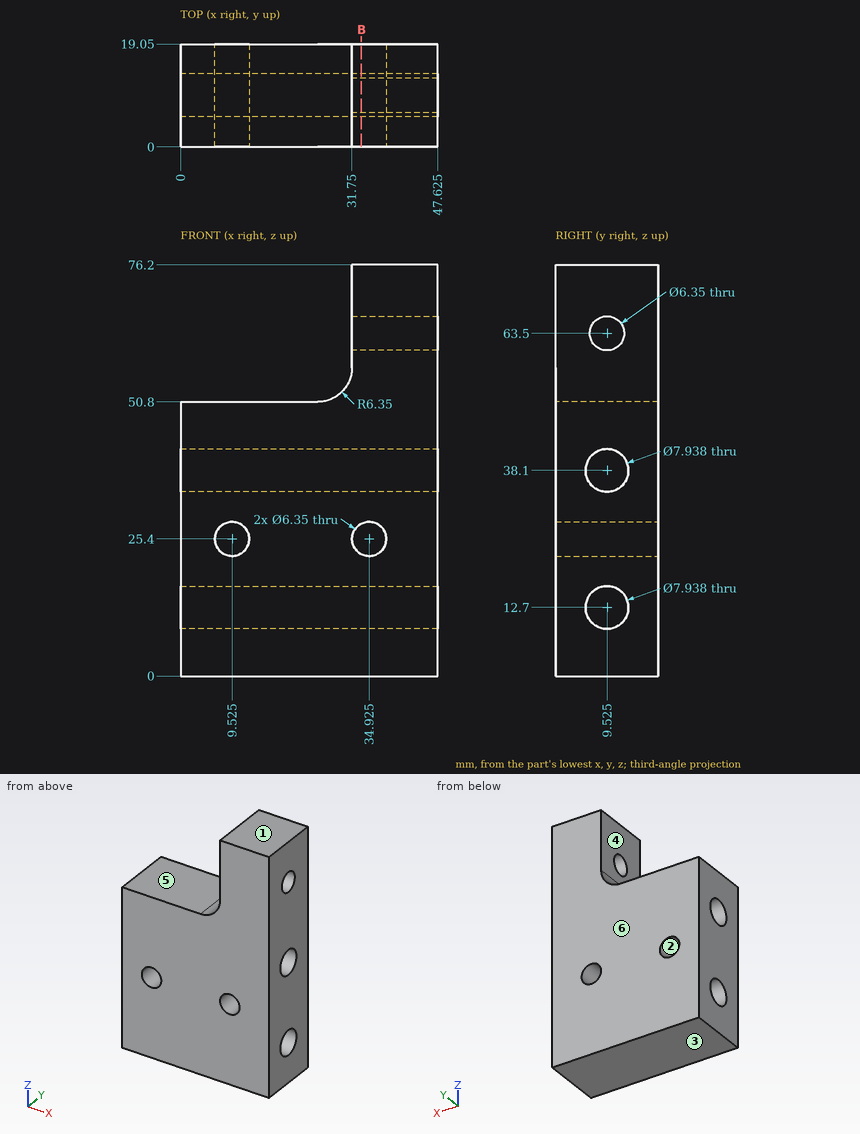
Design review of the part shown in the three views and the two pictorial views. Dimensions are in mm from the part's minimum x, y and z. A direction names the side the tool comes from. Round coordinates to 2 decimals unless told otherwise and drop trailing zeros.
(1) Mouldability with a two-part tool opening along Z and no side actions: class the marked faces 1, 2, 3 and 4 as released by +Z, released by -Z, zero draft, split by the parting line, or undercut.
Working result:
face 1: released by +Z
face 2: undercut
face 3: released by -Z
face 4: zero draft
(2) Wall thickness on L1, parallel to Y at x = 28, z = 38.1; L2, parallel to Z at x = 8.5, y = 11.25 (1 decimal); L3, parallel to Z at x = 26, y = 10: over which ranges is each line inside the solid? List them lowest first.
Working result:
L1: y = 0 to 5.56, 13.49 to 19.05
L2: z = 0 to 9.1, 16.3 to 22.4, 28.4 to 34.5, 41.7 to 50.8
L3: z = 0 to 8.76, 16.64 to 34.16, 42.04 to 50.83
(3) Take a section at B-B, the plane x = 33.5. Count the separate pieces of the cut face and the enclosed holes in it, plus the area to 3 significant figures.
Working result:
separate pieces: 2
enclosed holes: 3
area: 1,210 mm2
(4) For P1, Ø9, axis at y = 9.525, z = 38.1, coming from the -X side; P2, Ø7, axis at y = 9.525, z = 12.7, coming from the +X side, all flat-tipped, find the tip position at first contact; note any pin that passes through.
Working result:
P1: stops at x = 0
P2: passes through
(5) Tool access review of the marked faces 5 and 6: name each direction out of +Z, -Z, +X, -X, +Y, -Y from which nothing blocks a thin tool from reaching the whole face with its end or side.
Working result:
face 5: +Z, -X, +Y, -Y
face 6: +Z, -Z, +X, -X, +Y
